Read the model definition and answer for the solid it produces. Units are mm, in the model's axes. A direction names the side the tool comes from. Round coordinates to 2 decimals unless told otherwise and drop trailing zeros. Loops run counter-clockwise (first coordinate to the right, second up) from the corner with the lowest first, then second, coordinate; pieces in that order, holes last. Notation, with made-up numbers: (32.5, 48) - (66.5, 48) arc R20 cw to (66.5, 78) - close; hole circle Ø6 at (-40, -14). An arc over 180 degrees is marked (long way). Use CSV: the item, a comma, the result in double quotes. Start each with the question number.
1. Given pin 1 Ø8 at (x, y) = (-17, 17) entering from +Z; pin 2 Ø7 at (x, y) = (-17, 17) entering from -Z, each flat-ended and moving along its own axis, determine where each tip first touches the part or whether it passes through.
2. Find section D-D (z = 31). Give the vertices of the cut face in (x, y), and give its area (3 significant figures).
3. A tool of negligible diameter and unlimited length cuts with its end or side. For faces 1 (the cylindrical face through (13.68, -13.96, 111.45)), 2 (the cylindrical face through (20.479, 0.2, 105.546)), 3 (the flat face through (17, -20, 7)), 4 (the cylindrical face through (-3.47, -15.62, 56.79)), from which of +Z, -Z, +X, -X, +Y, -Y can it reach the whole face along a straight path? Write none if from no direction.
4. Consider line 1 along X through (y, z) = (-17, 74); line 2 along Y through (x, z) = (-17, 110); line 3 along Z through (x, y) = (8, 8). Determine where each line is inside the solid, lowest interval first.
5. Find section A-A (z = 14). Give the vertices of the cut face in (x, y).
6. Determine the mould class of faces 5 (the flat face through (0, 10, 115)), 6 (the flat face through (-17, -20, 108)), 7 (the flat face through (0, -22.5, 57)), 8 (the cylindrical face through (-20.32, -13.96, 3.45)) for opening direction Y: +Y half, -Y half, draft (parallel to the pull), parting line (faces both ways), or undercut.
7. Find section B-B (x = 0). Give the vertices of the cut face in (y, z).
8. Find section C-C (y = 0). Give the vertices of the cut face in (x, z), and give its area (3 significant figures).
from build123d import *

# Parameters (mm, degrees)
SKETCH1_W                                      = 45
SKETCH1_H                                      = 45
SKETCH1_R                                      = 2.75
SKETCH1_R_2                                    = 16
SMC_45_MM_SQUARE_BODY_AND_FOUR_5_5_MM_TH_DEPTH = 115
SKETCH2_R                                      = 16
HEAD_END_CLEARANCE_ENVELOPE_DEPTH              = 7
ROD_START                                      = 108
SKETCH3_R                                      = 16
SKETCH3_R_2                                    = 8.1
ROD_COVER_AND_16_MM_ROD_CLEARANCE_DEPTH        = 7
SKETCH4_R                                      = 4.5
REAR_BOLT_HEAD_COUNTERBORES_DEPTH              = 7
FRONT_START                                    = 108
SKETCH5_R                                      = 4.5
FRONT_MOUNTING_COUNTERBORES_DEPTH              = 7
TOP_START                                      = 22.5
SKETCH6_R                                      = 4.55
TOP_RC_1_8_PORT_CLEARANCE_FOR_LAYOUT_DEPTH     = 4.1


with BuildPart() as part:
    # Sketch1 → SMC 45 mm square body and four 5.5 mm through holes (new body)
    with BuildSketch(Plane.XY):
        Rectangle(SKETCH1_W, SKETCH1_H)
        with Locations((-17, -17)):
            Circle(SKETCH1_R, mode=Mode.SUBTRACT)
        with Locations((-17, 17)):
            Circle(SKETCH1_R, mode=Mode.SUBTRACT)
        with Locations((17, -17)):
            Circle(SKETCH1_R, mode=Mode.SUBTRACT)
        with Locations((17, 17)):
            Circle(SKETCH1_R, mode=Mode.SUBTRACT)
        Circle(SKETCH1_R_2, mode=Mode.SUBTRACT)
    extrude(amount=SMC_45_MM_SQUARE_BODY_AND_FOUR_5_5_MM_TH_DEPTH)

    # Sketch2 → Head end clearance envelope (add)
    with BuildSketch(Plane.XY):
        Circle(SKETCH2_R)
    extrude(amount=HEAD_END_CLEARANCE_ENVELOPE_DEPTH)

    # Sketch3 → Rod cover and 16 mm rod clearance (add)
    with BuildSketch(Plane.XY.offset(ROD_START)):
        Circle(SKETCH3_R)
        Circle(SKETCH3_R_2, mode=Mode.SUBTRACT)
    extrude(amount=ROD_COVER_AND_16_MM_ROD_CLEARANCE_DEPTH)

    # Sketch4 → Rear bolt head counterbores (cut)
    with BuildSketch(Plane.XY):
        with Locations((-17, -17)):
            Circle(SKETCH4_R)
        with Locations((-17, 17)):
            Circle(SKETCH4_R)
        with Locations((17, -17)):
            Circle(SKETCH4_R)
        with Locations((17, 17)):
            Circle(SKETCH4_R)
    extrude(amount=REAR_BOLT_HEAD_COUNTERBORES_DEPTH, mode=Mode.SUBTRACT)

    # Sketch5 → Front mounting counterbores (cut)
    with BuildSketch(Plane.XY.offset(FRONT_START)):
        with Locations((-17, -17)):
            Circle(SKETCH5_R)
        with Locations((-17, 17)):
            Circle(SKETCH5_R)
        with Locations((17, -17)):
            Circle(SKETCH5_R)
        with Locations((17, 17)):
            Circle(SKETCH5_R)
    extrude(amount=FRONT_MOUNTING_COUNTERBORES_DEPTH, mode=Mode.SUBTRACT)

    # Sketch6 → Top Rc 1/8 port clearance for layout (cut)
    with BuildSketch(Plane(origin=(0, 0, 0), x_dir=(0, 0, -1), z_dir=(1, 0, 0)).offset(TOP_START)):
        with Locations((-14, 0)):
            Circle(SKETCH6_R)
        with Locations((-101, 0)):
            Circle(SKETCH6_R)
    extrude(amount=-TOP_RC_1_8_PORT_CLEARANCE_FOR_LAYOUT_DEPTH, mode=Mode.SUBTRACT)


solid = part.part
Filled sheet:
1,pin 1,"stops at z = 108"
1,pin 2,"stops at z = 7"
2,outline,"(-22.5, -22.5) - (22.5, -22.5) - (22.5, 22.5) - (-22.5, 22.5) - close; hole circle Ø5.5 at (-17, -17); hole circle Ø5.5 at (-17, 17); hole circle Ø32 at (0, 0); hole circle Ø5.5 at (17, -17); hole circle Ø5.5 at (17, 17)"
2,area,"1,130 mm²"
3,face 1,"+Z"
3,face 2,"+X"
3,face 3,"-Z"
3,face 4,"none"
4,line 1,"x = -22.5 to -19.75, -14.25 to 14.25, 19.75 to 22.5"
4,line 2,"y = -22.5 to -21.5, -12.5 to 12.5, 21.5 to 22.5"
4,line 3,"z = 0 to 7, 108 to 115"
5,outline,"(-22.5, -22.5) - (22.5, -22.5) - (22.5, -4.55) - (18.4, -4.55) - (18.4, 4.55) - (22.5, 4.55) - (22.5, 22.5) - (-22.5, 22.5) - close; hole circle Ø5.5 at (-17, -17); hole circle Ø5.5 at (-17, 17); hole circle Ø32 at (0, 0); hole circle Ø5.5 at (17, -17); hole circle Ø5.5 at (17, 17)"
6,face 5,"draft"
6,face 6,"undercut"
6,face 7,"-Y half"
6,face 8,"undercut"
7,outline,"(-22.5, 0) - (22.5, 0) - (22.5, 115) - (8.1, 115) - (8.1, 108) - (16, 108) - (16, 7) - (-16, 7) - (-16, 108) - (-8.1, 108) - (-8.1, 115) - (-22.5, 115) - close"
8,outline,"(-22.5, 0) - (22.5, 0) - (22.5, 9.45) - (18.4, 9.45) - (18.4, 18.55) - (22.5, 18.55) - (22.5, 96.45) - (18.4, 96.45) - (18.4, 105.55) - (22.5, 105.55) - (22.5, 115) - (8.1, 115) - (8.1, 108) - (16, 108) - (16, 7) - (-16, 7) - (-16, 108) - (-8.1, 108) - (-8.1, 115) - (-22.5, 115) - close"
8,area,"1,750 mm²"
